Here's the drawing with two shaded views (mm, measured from the low corner). I have some questions. Coordinates: 2 decimals unless noted, no trailing zeros. Write each loop counter-clockwise with the first axis right and the second up, starting at its lowest first coordinate (ties: lowest second). Pieces come first, ordered by that corner, then holes. Notation, with made-up numbers: (14.5, -25) -> (21.5, -25) arc R17 ccw to (21.5, -14) -> close; hole circle Ø4 at (-19, 36). An arc over 180 degrees is marked (long way). Put each result on its own line as item: value.
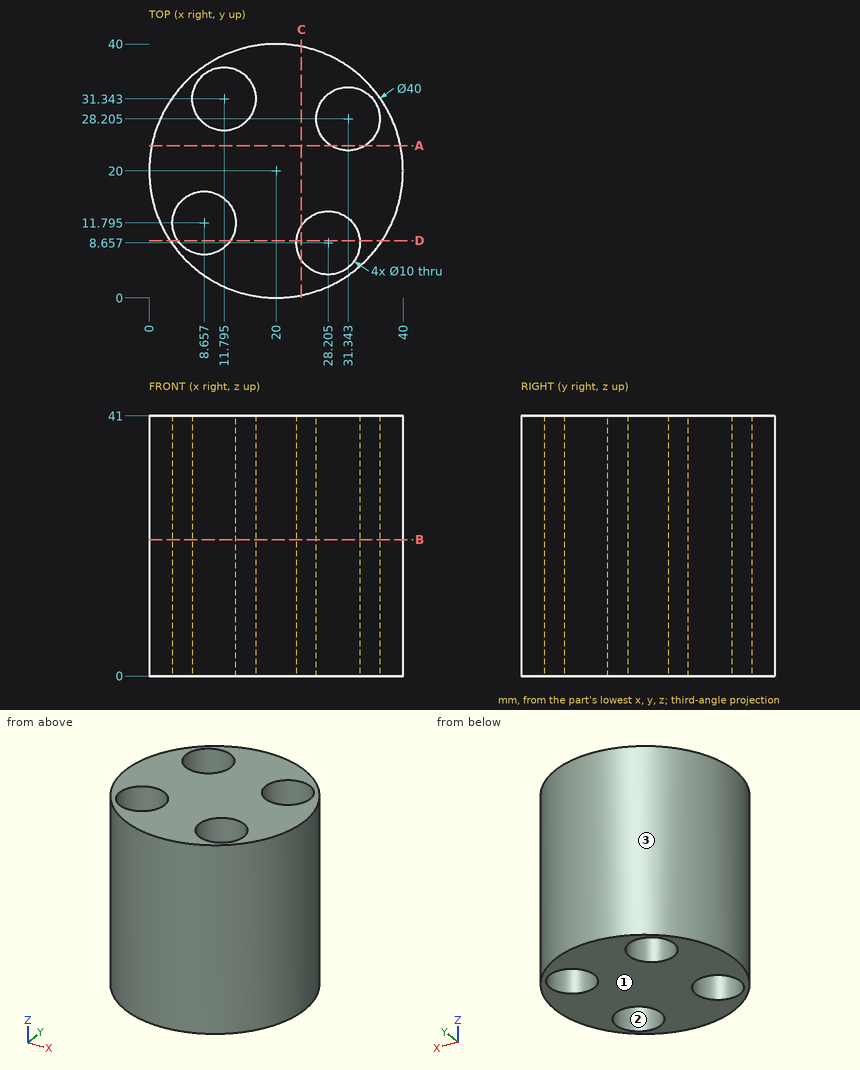
Item 1: For P1, Ø6, axis at x = 29, z = 25, coming from the +Y side; P2, Ø2, axis at y = 7.5, z = 7.5, coming from the +X side; P3, Ø6, axis at x = 28.21, y = 8.66, coming from the +Z side; P4, Ø8, axis at x = 9, y = 32, coming from the -Z side, each with a flat end and sliding along its axis, tell me the tip position at first contact or that it passes through.
Output:
P1: stops at y = 39.08
P2: stops at x = 36.36
P3: passes through
P4: stops at z = 0
Item 2: Imagine slicing it at B-B on z = 21.5. Write out the boundary of the cut face in (x, y) (1 decimal).
Output:
outline: circle Ø40 at (20, 20); hole circle Ø10 at (8.7, 11.8); hole circle Ø10 at (11.8, 31.3); hole circle Ø10 at (28.2, 8.7); hole circle Ø10 at (31.3, 28.2)
Item 3: Please list where these lines run through material, in increasing order: line 1 along Y through (x, z) = (9.5, 23) (1 decimal); line 2 along X through (y, z) = (13, 29) (1 decimal); line 3 along X through (y, z) = (11, 29.5). Write a range as from..to.
Output:
line 1: y = 3..6.9, 16.7..26.9, 35.8..37
line 2: x = 1.3..3.8, 13.5..25.7, 30.7..38.7
line 3: x = 2.14..3.72, 13.59..23.79, 32.62..37.86
Item 4: Imagine slicing it at C-C on x = 24. Write out the boundary of the cut face in (y, z), then the cut area to 4 significant figures.
Output:
outline: (0.4, 0) -> (5.95, 0) -> (5.95, 41) -> (0.4, 41) -> close; (11.36, 0) -> (39.6, 0) -> (39.6, 41) -> (11.36, 41) -> close
area: 1,385 mm²
Item 5: Imagine slicing it at A-A on y = 24. Write out the boundary of the cut face in (x, z).
Output:
outline: (0.4, 0) -> (28.64, 0) -> (28.64, 41) -> (0.4, 41) -> close; (34.05, 0) -> (39.6, 0) -> (39.6, 41) -> (34.05, 41) -> close
Item 6: Imagine slicing it at D-D on y = 9. Write out the boundary of the cut face in (x, z).
Output:
outline: (3.3, 0) -> (4.51, 0) -> (4.51, 41) -> (3.3, 41) -> close; (12.8, 0) -> (23.22, 0) -> (23.22, 41) -> (12.8, 41) -> close; (33.19, 0) -> (36.7, 0) -> (36.7, 41) -> (33.19, 41) -> close
Item 7: If we mould it in two halves opening along Y, with no side actions, what happens to the marked faces 1, 2 and 3? For each: released by +Y, released by -Y, zero draft, split by the parting line, or undercut.
Output:
face 1: zero draft
face 2: undercut
face 3: split by the parting line
